The model under review builds one solid part; all positions refer to its coordinate system, in mm. Face numbers are marked on the shaded views. A direction names the side the tool comes from. Coordinates: 2 decimals unless noted, no trailing zeros. Loops run counter-clockwise (first coordinate to the right, second up) from the corner with the lowest first, then second, coordinate; pieces in that order, holes last. Notation, with made-up numbers: M 81,-1 L 126,-1 A15 cw 126,6 Z; hole C 20.5,-3.75 d8. An arc over 180 degrees is marked long. One line per item, written item: value.
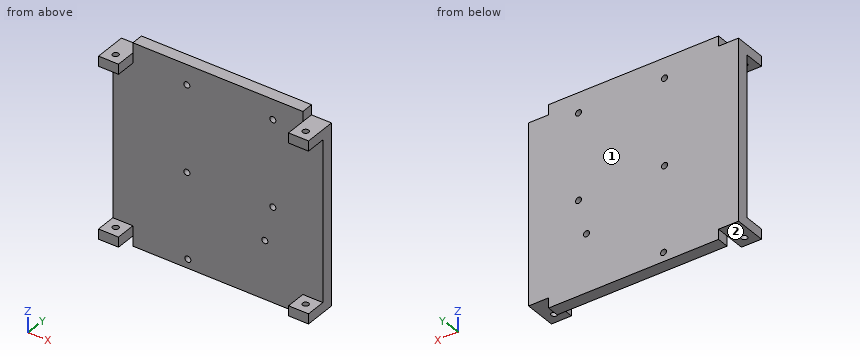
```python
from build123d import *

# Parameters (mm, degrees)
SKETCH1_W           = 105
SKETCH1_H           = 100
BOSS_EXTRUDE1_DEPTH = 6
SKETCH2_W           = 10
SKETCH2_H           = 5
CUT_EXTRUDE1_DEPTH  = 10
SKETCH3_W           = 10
SKETCH3_H           = 5
BOSS_EXTRUDE2_DEPTH = 10
SKETCH4_R           = 1.5
CUT_EXTRUDE2_DEPTH  = 142.950695666
SKETCH5_R           = 1.5
CUT_EXTRUDE4_DEPTH  = 6
SKETCH6_R           = 1.5
CUT_EXTRUDE5_DEPTH  = 6


with BuildPart() as part:
    # Sketch1 → Boss-Extrude1 (new body)
    with BuildSketch(Plane(origin=(0, 0, 0), x_dir=(1, 0, 0), z_dir=(0, 1, 0))):
        with Locations((52.5, 50)):
            Rectangle(SKETCH1_W, SKETCH1_H)
    extrude(amount=BOSS_EXTRUDE1_DEPTH)

    # Sketch2 → Cut-Extrude1 (cut)
    with BuildSketch(Plane.XZ):
        with Locations((100, -97.5)):
            Rectangle(SKETCH2_W, SKETCH2_H)
        with Locations((5, -97.5)):
            Rectangle(SKETCH2_W, SKETCH2_H)
        with Locations((100, -2.5)):
            Rectangle(SKETCH2_W, SKETCH2_H)
        with Locations((5, -2.5)):
            Rectangle(SKETCH2_W, SKETCH2_H)
    extrude(amount=-CUT_EXTRUDE1_DEPTH, mode=Mode.SUBTRACT)

    # Sketch3 → Boss-Extrude2 (add)
    with BuildSketch(Plane(origin=(0, 0, 0), x_dir=(-1, 0, 0), z_dir=(0, -1, 0))):
        with Locations((-100, 92.5)):
            Rectangle(SKETCH3_W, SKETCH3_H)
        with Locations((-100, 7.5)):
            Rectangle(SKETCH3_W, SKETCH3_H)
        with Locations((-5, 7.5)):
            Rectangle(SKETCH3_W, SKETCH3_H)
        with Locations((-5, 92.5)):
            Rectangle(SKETCH3_W, SKETCH3_H)
    extrude(amount=BOSS_EXTRUDE2_DEPTH)

    # Sketch4 → Cut-Extrude2 (cut, through all)
    with BuildSketch(Plane(origin=(0, 0, -95), x_dir=(-1, 0, 0), z_dir=(0, 0, -1))):
        with Locations((-100, -5)):
            Circle(SKETCH4_R)
        with Locations((-5, -5)):
            Circle(SKETCH4_R)
    extrude(amount=-CUT_EXTRUDE2_DEPTH, mode=Mode.SUBTRACT)

    # Sketch5 → Cut-Extrude4 (cut)
    with BuildSketch(Plane(origin=(0, 0, 0), x_dir=(-1, 0, 0), z_dir=(0, -1, 0))):
        with Locations(Location((-37, 10, 0), (0, 0, 90))):
            Circle(SKETCH5_R)
        with Locations(Location((-37, 53, 0), (0, 0, 90))):
            Circle(SKETCH5_R)
        with Locations(Location((-80, 53, 0), (0, 0, 90))):
            Circle(SKETCH5_R)
        with Locations(Location((-80, 10, 0), (0, 0, 90))):
            Circle(SKETCH5_R)
    extrude(amount=-CUT_EXTRUDE4_DEPTH, mode=Mode.SUBTRACT)

    # Sketch6 → Cut-Extrude5 (cut)
    with BuildSketch(Plane(origin=(0, 0, 0), x_dir=(-1, 0, 0), z_dir=(0, -1, 0))):
        with Locations(Location((-37.5, 95.5, 0), (0, 0, 90))):
            Circle(SKETCH6_R)
        with Locations(Location((-76, 71, 0), (0, 0, 90))):
            Circle(SKETCH6_R)
    extrude(amount=-CUT_EXTRUDE5_DEPTH, mode=Mode.SUBTRACT)


solid = part.part
```
(1) Add section A-A on x = 76. State the section outline as (y, z) points, then the cut area to 3 significant figures.
Checks:
outline: M 0,-100 L 6,-100 L 6,-72.5 L 0,-72.5 Z; M 0,-69.5 L 6,-69.5 L 6,0 L 0,0 Z
area: 582 mm^2
(2) Add section D-D on x = 100. State the section outline as (y, z) points, then the cut area to 3 significant figures.
Checks:
outline: M -10,-95 L -6.5,-95 L -6.5,-90 L -10,-90 Z; M -10,-10 L -6.5,-10 L -6.5,-5 L -10,-5 Z; M -3.5,-95 L 6,-95 L 6,-5 L -3.5,-5 L -3.5,-10 L 0,-10 L 0,-90 L -3.5,-90 Z
area: 610 mm^2
(3) Tool access review of the marked faces 1 and 2: name each direction out of +Z, -Z, +X, -X, +Y, -Y from which nothing blocks a thin tool from reaching the whole face with its end or side.
Checks:
face 1: +Z, -Z, +X, -X, +Y
face 2: -Z, -X, +Y, -Y
(4) Insertion check: pin 1 Ø2.5 at (y, z) = (4.5, -1.5) entering from +X; pin 2 Ø3.5 at (x, z) = (80, -53) entering from +Y; pin 3 Ø10 at (x, z) = (50, -87.5) entering from -Y; pin 4 Ø8 at (x, y) = (99, -4.5) entering from -Z. Each pin has a flat end and moves straight along its axis. Give the tip position at first contact, or say it passes through.
Checks:
pin 1: x = 95
pin 2: y = 6
pin 3: y = 0
pin 4: z = -95
(5) To check wall thickness, follow L1, parallel to X at y = -4.75, z = -8; L2, parallel to X at y = 2.9, z = -53; L3, parallel to X at y = 1.3, z = -71. State the ranges of each line that lie inside material, in increasing order. Write a range as [from, to].
Checks:
L1: [0, 3.52], [6.48, 10], [95, 98.52], [101.48, 105]
L2: [0, 35.5], [38.5, 78.5], [81.5, 105]
L3: [0, 74.5], [77.5, 105]
(6) Add section C-C on z = -53. State the section outline as (x, y) points, then the cut area to 3 significant figures.
Checks:
outline: M 0,0 L 35.5,0 L 35.5,6 L 0,6 Z; M 38.5,0 L 78.5,0 L 78.5,6 L 38.5,6 Z; M 81.5,0 L 105,0 L 105,6 L 81.5,6 Z
area: 594 mm^2
(7) Add section B-B on y = 4. State the section outline as (x, z) points, then the cut area to 3 significant figures.
Checks:
outline: M 0,-95 L 10,-95 L 10,-100 L 95,-100 L 95,-95 L 105,-95 L 105,-5 L 95,-5 L 95,0 L 10,0 L 10,-5 L 0,-5 Z; hole C 37,-53 d3; hole C 37,-10 d3; hole C 37.5,-95.5 d3; hole C 76,-71 d3; hole C 80,-53 d3; hole C 80,-10 d3
area: 10,300 mm^2
